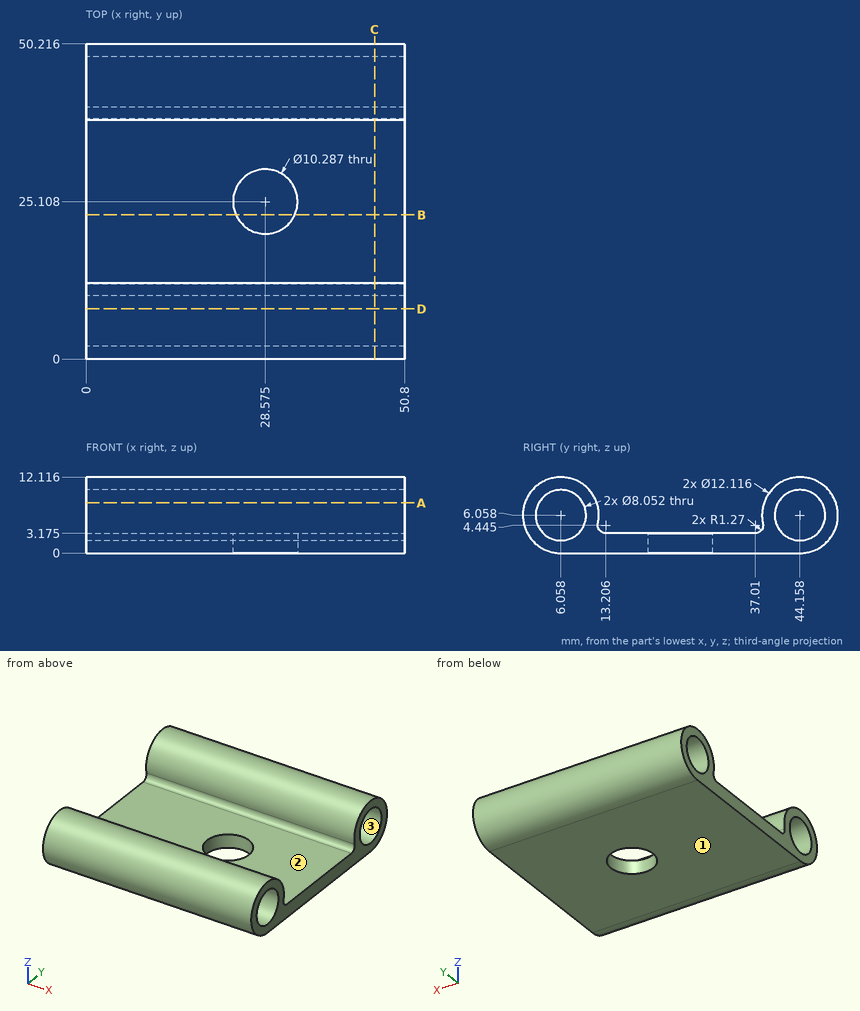
Geometry: see drawing. Coordinates: mm, zero at the bounding-box minimum. Coordinates: 2 decimals unless noted, no trailing zeros. Order: outer loops, then holes, each group sorted by start corner. A loop starts at its lowest first (then second) coordinate and runs counter-clockwise, first axis right, second up. Notation, with made-up numbers: M 85.5,-31.5 L 106.5,-31.5 A24 ccw 106.5,5.5 Z; hole C 24,4 d6. An arc over 180 degrees is marked long. Write item = value, one per line. Start each with the question number.
(1) Section C-C on x = 46. Output: boundary loops of the cut face in (y, z) (1 decimal), and give its area (3 significant figures).
(2) Section D-D on y = 8. Output: boundary loops of the cut face in (x, z), and give its area (3 significant figures).
(3) First-contact query: P1, Ø12, axis at x = 31, y = 20, coming from the +Z side (3 decimals); P2, Ø2, axis at x = 13.5, z = 9.5, coming from the -Y side; P3, Ø6, axis at x = 36, z = 10.5, coming from the -Y side. Flat tips, straight axial feed; report the tip coordinate or a pass-through.
(4) Line query: line 1 along X through (y, z) = (25, 1.25); line 2 along Y through (x, z) = (46, 5.5) (1 decimal); line 3 along Y through (x, z) = (49, 9.5) (1 decimal). Output: solid intervals per line, ascending. Write a range as [from, to].
(5) Pull-direction query (Z, two-part tool) for the marked faces 1, 2 and 3; classes: released by +Z, released by -Z, zero draft, split by the parting line, or undercut.
(6) Section B-B on y = 23. Output: boundary loops of the cut face in (x, z) (1 decimal).
(7) Section A-A on z = 8. Output: boundary loops of the cut face in (x, y).
Result set:
q1.outline = M 6.1,0 L 44.2,0 A6.1 ccw long 38.2,4.7 A1.3 cw 37,3.2 L 13.2,3.2 A1.3 cw 12,4.7 A6.1 ccw long Z; hole C 6.1,6.1 d8.1; hole C 44.2,6.1 d8.1
q1.area = 227 mm²
q2.outline = M 0,0 L 50.8,0 L 50.8,2.53 L 0,2.53 Z; M 0,9.58 L 50.8,9.58 L 50.8,11.8 L 0,11.8 Z
q2.area = 241 mm²
q3.P1 = 3.175
q3.P2 = 0.51
q3.P3 = 0.17
q4.line_1 = [0, 23.43], [33.72, 50.8]
q4.line_2 = [0, 2.1], [10, 12.1], [38.1, 40.2], [48.1, 50.2]
q4.line_3 = [1.1, 4], [8.1, 11], [39.2, 42.1], [46.2, 49.1]
q5.face_1 = released by -Z
q5.face_2 = released by +Z
q5.face_3 = undercut
q6.outline = M 0,0 L 23.9,0 L 23.9,3.2 L 0,3.2 Z; M 33.3,0 L 50.8,0 L 50.8,3.2 L 33.3,3.2 Z
q7.outline = M 0,0.32 L 50.8,0.32 L 50.8,2.53 L 0,2.53 Z; M 0,9.58 L 50.8,9.58 L 50.8,11.8 L 0,11.8 Z; M 0,38.42 L 50.8,38.42 L 50.8,40.63 L 0,40.63 Z; M 0,47.68 L 50.8,47.68 L 50.8,49.9 L 0,49.9 Z
